Verification items for the finished model (mm, model axes). Face numbers are marked on the shaded views. A direction names the side the tool comes from. Round coordinates to 2 decimals unless told otherwise and drop trailing zeros. Loops run counter-clockwise (first coordinate to the right, second up) from the corner with the lowest first, then second, coordinate; pieces in that order, holes last. Notation, with made-up numbers: M 60.25,79 L 99.25,79 A16 ccw 99.25,107 Z; hole C 38.5,62 d4. An arc over 180 degrees is marked long. Answer as CSV lines item,"result".
```python
from build123d import *

# Parameters (mm, degrees)
BOSS_EXTRUDE1_DEPTH     = 17
CUT_EXTRUDE1_REACH      = 46.598
SKETCH3_W               = 35
SKETCH3_H               = 14
FILLET1_R               = 5
M3_CLEARANCE_HOLE1_D    = 3.6
CIRPATTERN1_START       = 14
CIRPATTERN1_DEPTH       = 3
CIRPATTERN1_START_2     = 6.8000001
CIRPATTERN1_2_DEPTH     = 7.1999999
CIRPATTERN1_3_DEPTH     = 6.8000001
CIRPATTERN1_START_3     = -40
CIRPATTERN1_4_OUTLINE_R = 1.8
CIRPATTERN1_4_DEPTH     = 5
CIRPATTERN1_START_4     = 35
CIRPATTERN1_5_OUTLINE_R = 1.8
CIRPATTERN1_5_DEPTH     = 5
SKETCH6_R               = 50
BOSS_EXTRUDE2_DEPTH     = 3
FILLET6_R               = 2


with BuildPart() as part:
    # Sketch2 → Boss-Extrude1 (new body)
    with BuildSketch(Plane(origin=(0, 0, 0), x_dir=(1, 0, 0), z_dir=(0, 1, 0))):
        Polygon((0, 0), (-5, 2.886751346), (-5, 40), (5, 40), (5, 2.886751346), align=None)
    extrude(amount=BOSS_EXTRUDE1_DEPTH)

    # Sketch3 → Cut-Extrude1 (cut, up to next)
    with BuildSketch(Plane(origin=(5, 0, 0), x_dir=(0, 0, -1), z_dir=(1, 0, 0)), mode=Mode.PRIVATE) as cut_extrude1_sk1:
        with Locations((17.5, 7)):
            Rectangle(SKETCH3_W, SKETCH3_H)
    cut_extrude1_tool1 = extrude(cut_extrude1_sk1.sketch, amount=-CUT_EXTRUDE1_REACH, mode=Mode.PRIVATE) & part.part
    add(cut_extrude1_tool1.solids().sort_by_distance((5, 7, -17.5))[0], mode=Mode.SUBTRACT)

    # Fillet1
    fillet1_edges = [part.edges().sort_by_distance(p)[0] for p in [
        (-5, 0, -37.5),
        (5, 0, -37.5),
    ]]
    fillet(fillet1_edges, radius=FILLET1_R - 0.0001)  # a hair under: the kernel refuses the full size

    # M3 Clearance Hole1 (through all)
    with Locations(Plane(origin=(0, 0, -40), x_dir=(-1, 0, 0), z_dir=(0, 0, -1))):
        with Locations((0, 5)):
            Hole(M3_CLEARANCE_HOLE1_D / 2)

    # CirPattern1: read off the stored shape, not the designer's step
    # CirPattern1 outline → CirPattern1 (add)
    with BuildSketch(Plane(origin=(0, 0, 0), x_dir=(1, 0, 0), z_dir=(0, 1, 0)).offset(CIRPATTERN1_START)):
        Polygon((-37.141016151, -15.669872981), (-32.141016151, -24.330127019), (0, -5.773502692), (32.141016151, -24.330127019), (37.141016151, -15.669872981), (5, 2.886751346), (0, 0), (-5, 2.886751346), align=None)
    extrude(amount=CIRPATTERN1_DEPTH)

    # CirPattern1 2 outline → CirPattern1 2 (add)
    with BuildSketch(Plane(origin=(0, 0, 0), x_dir=(1, 0, 0), z_dir=(0, 1, 0)).offset(CIRPATTERN1_START_2)):
        Polygon((-32.810889132, -13.169872981), (-37.141016151, -15.669872981), (-32.141016151, -24.330127019), (-27.810889132, -21.830127019), align=None)
        Polygon((32.810889132, -13.169872981), (27.810889132, -21.830127019), (32.141016151, -24.330127019), (37.141016151, -15.669872981), align=None)
    extrude(amount=CIRPATTERN1_2_DEPTH)

    # CirPattern1 3 outline → CirPattern1 3 (add)
    with BuildSketch(Plane(origin=(0, 0, 0), x_dir=(1, 0, 0), z_dir=(0, 1, 0))):
        Polygon((32.810889132, -13.169872981), (27.810889132, -21.830127019), (32.141016151, -24.330127019), (37.141016151, -15.669872981), align=None)
        Polygon((-32.810889132, -13.169872981), (-37.141016151, -15.669872981), (-32.141016151, -24.330127019), (-27.810889132, -21.830127019), align=None)
    extrude(amount=CIRPATTERN1_3_DEPTH)

    # CirPattern1 4 outline → CirPattern1 4 (cut)
    with BuildSketch(Plane(origin=(0, 0, 0), x_dir=(0.500000000000006, 0, 0.8660254037844353), z_dir=(0.8660254037844352, 0, -0.5000000000000061)).offset(CIRPATTERN1_START_3)):
        with BuildLine():
            Line((5, 0), (0, 0))
            ThreePointArc((0, 0), (3.535533906, -1.464466094), (5, -5))
            Line((5, -5), (5, 0))
        make_face()
        with BuildLine():
            ThreePointArc((-5, -5), (-3.535533906, -1.464466094), (0, 0))
            Line((0, 0), (-5, 0))
            Line((-5, 0), (-5, -5))
        make_face()
        with Locations((0, -5)):
            Circle(CIRPATTERN1_4_OUTLINE_R)
    extrude(amount=CIRPATTERN1_4_DEPTH, mode=Mode.SUBTRACT)

    # CirPattern1 5 outline → CirPattern1 5 (cut)
    with BuildSketch(Plane(origin=(0, 0, 0), x_dir=(0.4999999999999894, 0, -0.8660254037844448), z_dir=(0.8660254037844447, 0, 0.4999999999999898)).offset(CIRPATTERN1_START_4)):
        with BuildLine():
            Line((-5, 0), (0, 0))
            ThreePointArc((0, 0), (-3.535533906, 1.464466094), (-5, 5))
            Line((-5, 5), (-5, 0))
        make_face()
        with BuildLine():
            ThreePointArc((5, 5), (3.535533906, 1.464466094), (0, 0))
            Line((0, 0), (5, 0))
            Line((5, 0), (5, 5))
        make_face()
        with Locations((0, 5)):
            Circle(CIRPATTERN1_5_OUTLINE_R)
    extrude(amount=CIRPATTERN1_5_DEPTH, mode=Mode.SUBTRACT)

    # Sketch6 → Boss-Extrude2 (add)
    with BuildSketch(Plane(origin=(0, 14, 0), x_dir=(1, 0, 0), z_dir=(0, 1, 0))):
        with Locations(Location((0, 0, 0), (0, 0, 90))):
            Circle(SKETCH6_R)
    extrude(amount=BOSS_EXTRUDE2_DEPTH)

    # Fillet6
    fillet6_edges = [part.edges().sort_by_distance(p)[0] for p in [
        (5, 14, -37.5),
        (0, 14, -40),
        (-5, 14, -37.5),
        (-34.975952642, 14, 14.419872981),
        (-34.641016151, 14, 20),
        (-29.975952642, 14, 23.080127019),
        (29.975952642, 14, 23.080127019),
        (34.641016151, 14, 20),
        (34.975952642, 14, 14.419872981),
        (0, 14, -35),
        (-30.310889132, 14, 17.5),
        (30.310889132, 14, 17.5),
    ]]
    fillet(fillet6_edges, radius=FILLET6_R)


solid = part.part
```
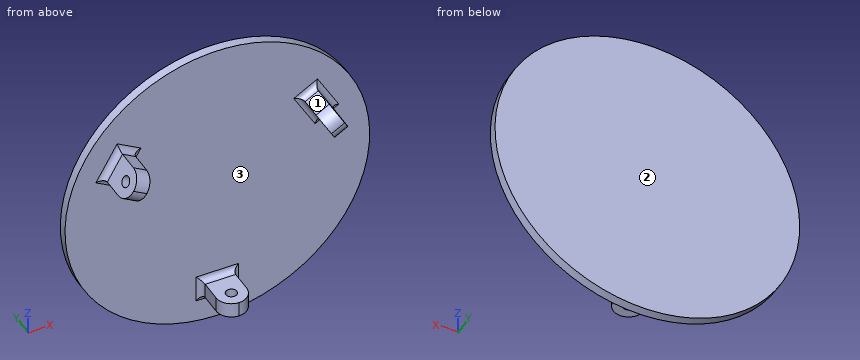
1) Section check A-A (y = 10.5). Record the cut outline in (x, z), plus the area to 3 significant figures.
Here are the results:
outline,"M -37.14,15.67 L -32.81,13.17 L -27.81,21.83 L -32.14,24.33 Z; M -5,-40 L 5,-40 L 5,-35 L -5,-35 Z; M 27.81,21.83 L 32.81,13.17 L 37.14,15.67 L 32.14,24.33 Z"
area,"150 mm^2"
2) Section check C-C (z = 1). Record the cut outline in (x, y).
Here are the results:
outline,"M -49.99,14 L 49.99,14 L 49.99,17 L -49.99,17 Z"
3) Go/stop test with flat-tipped pins: pin 1 (5 mm diameter, centred on x = -2.5, y = 8, fed in from +Z); pin 2 (1 mm diameter, centred on y = 8, z = 22.5, fed in from +X); pin 3 (1 mm diameter, centred on x = 12.5, z = -22.5, fed in from -Y). Record where each tip stops, or that it passes through.
Here are the results:
pin 1,"stops at z = -35"
pin 2,"stops at x = 33.49"
pin 3,"stops at y = 14"
4) Set-up check for the marked faces 1, 2 and 3: record each of +Z, -Z, +X, -X, +Y, -Y from which the full face is reachable in a straight line by a thin tool's end or side.
Here are the results:
face 1,"+Z, -Y"
face 2,"+Z, -Z, +X, -X, +Y"
face 3,"-Y"
5) Section check B-B (y = 15.75). Record the cut outline in (x, z).
Here are the results:
outline,"C 0,0 d100"
6) Section check D-D (y = 2). Record the cut outline in (x, z).
Here are the results:
outline,"M -36.64,16.54 L -32.31,14.04 L -28.31,20.96 L -32.64,23.46 Z; M -4,-40 L 4,-40 L 4,-35 L -4,-35 Z; M 28.31,20.96 L 32.31,14.04 L 36.64,16.54 L 32.64,23.46 Z"
7) Material ranges on probe 1 along Y at (x, z) = (0, -38.7); probe 2 along Y at (x, z) = (-10, -11); probe 3 along Z at (x, y) = (-2.5, 5.5), recorded low to high.
Here are the results:
probe 1,"y = 0 to 3.2, 6.8 to 17"
probe 2,"y = 14 to 17"
probe 3,"z = -40 to -35"
